from build123d import *

# Parameters (mm, degrees)
SKETCH1_W               = 8
SKETCH1_H               = 8
BOSS_EXTRUDE1_DEPTH     = 3
CUT_EXTRUDE1_DEPTH      = 12.704699911
CUT_EXTRUDE1_DEPTH_BACK = 12.704699911
CUT_EXTRUDE2_DEPTH      = 11
SKETCH4_R               = 1.8
CUT_EXTRUDE3_DEPTH      = 0.8
SKETCH5_W               = 8
SKETCH5_H               = 1
BOSS_EXTRUDE2_DEPTH     = 2
FILLET1_R               = 4
CUT_EXTRUDE4_DEPTH      = 0.4
CUT_EXTRUDE5_DEPTH      = 0.4


with BuildPart() as part:
    # Sketch1 → Boss-Extrude1 (new body)
    with BuildSketch(Plane(origin=(0, 0, 0), x_dir=(1, 0, 0), z_dir=(0, 1, 0))):
        with Locations((4, 4)):
            Rectangle(SKETCH1_W, SKETCH1_H)
    extrude(amount=BOSS_EXTRUDE1_DEPTH)

    # Sketch2 → Cut-Extrude1 (cut, two sides: drawn at the far end of the back side and taken through both)
    with BuildSketch(Plane.XY.offset(-CUT_EXTRUDE1_DEPTH_BACK)):
        Polygon((0, 0), (0.6, 3), (0, 3), align=None)
        Polygon((8, 0), (7.4, 3), (8, 3), align=None)
    extrude(amount=CUT_EXTRUDE1_DEPTH + CUT_EXTRUDE1_DEPTH_BACK, mode=Mode.SUBTRACT)

    # Sketch3 → Cut-Extrude2 (cut)
    with BuildSketch(Plane(origin=(0, 0, 0), x_dir=(0, 0, -1), z_dir=(1, 0, 0))):
        Polygon((0, 0), (0.6, 3), (0, 3), align=None)
        Polygon((8, 3), (7.4, 3), (8, 0), align=None)
    extrude(amount=CUT_EXTRUDE2_DEPTH, mode=Mode.SUBTRACT)

    # Sketch4 → Cut-Extrude3 (cut)
    with BuildSketch(Plane.XZ):
        with Locations(Location((4, -3.75, 0), (0, 0, 270))):
            Circle(SKETCH4_R)
    extrude(amount=-CUT_EXTRUDE3_DEPTH, mode=Mode.SUBTRACT)

    # Sketch5 → Boss-Extrude2 (add)
    with BuildSketch(Plane.XZ):
        with Locations((4, -7.5)):
            Rectangle(SKETCH5_W, SKETCH5_H)
    extrude(amount=BOSS_EXTRUDE2_DEPTH)

    # Fillet1
    # the kernel refuses this fillet: 4 mm, written as the material it takes off along each edge
    with BuildSketch(Plane(origin=(8, -2, -16.660254038), x_dir=(0, 1, 0), z_dir=(0, 0, 1)), Plane(origin=(0, -2, 1.660254038), x_dir=(0, 1, 0), z_dir=(0, 0, -1))) as fillet1_piece_1:
        with BuildLine():
            CenterArc((4, 3.464101615), FILLET1_R, 180, 60)
            Line((0, 3.464101615), (-0.08, 3.464101615))
            Line((-0.08, 3.464101615), (-0.08, 0))
            Line((-0.08, 0), (0, -0.08))
            ThreePointArc((0, -0.08), (1, -0.08), (1.96, -0.069282032))
            Line((1.96, -0.069282032), (2, 0))
        make_face()
    extrude(amount=18.320508076, mode=Mode.SUBTRACT)

    # Sketch6 → Cut-Extrude4 (cut)
    with BuildSketch(Plane(origin=(0, 3, 0), x_dir=(1, 0, 0), z_dir=(0, 1, 0))):
        Polygon((2.721575188, 1.941169366), (2.721575188, 5.941169366), (5.439523906, 5.941169366), (5.439523906, 5.2745027), (3.490805957, 5.2745027), (3.490805957, 4.300143725), (5.18311365, 4.300143725), (5.18311365, 3.633477059), (3.490805957, 3.633477059), (3.490805957, 1.941169366), align=None)
    extrude(amount=-CUT_EXTRUDE4_DEPTH, mode=Mode.SUBTRACT)

    # Sketch7 → Cut-Extrude5 (cut)
    with BuildSketch(Plane(origin=(0, 3, 0), x_dir=(1, 0, 0), z_dir=(0, 1, 0))):
        Polygon((6.374503362, 0.955347226), (6.374503362, 3.239962611), (7.020657208, 3.239962611), (7.020657208, 2.939962611), (6.720657208, 2.939962611), (6.720657208, 1.255347226), (7.020657208, 1.255347226), (7.020657208, 0.955347226), align=None)
    extrude(amount=-CUT_EXTRUDE5_DEPTH, mode=Mode.SUBTRACT)


solid = part.part
Design review of the part built by this model. Coordinates are the model's own, in mm. A direction names the side the tool comes from. Coordinates: 2 decimals unless noted, no trailing zeros. Loops run counter-clockwise (first coordinate to the right, second up) from the corner with the lowest first, then second, coordinate; pieces in that order, holes last. Notation, with made-up numbers: (73, 11) -> (117, 11) arc R17 cw to (117, 23) -> close; hole circle Ø3 at (-21, 48.5). An arc over 180 degrees is marked (long way). Use a Markdown table: item, result. Add a question column.
Item 1: We need section D-D, the plane y = 0.95. Write out the cut boundary in (x, z).
Item 2: Wall thickness on L1, parallel to Z at x = 4.5, y = -0.2; L2, parallel to X at y = 0.35, z = -3.75; L3, parallel to Y at x = 7, z = -6.5: over which ranges is each line inside the solid? List them lowest first. Write a range as from..to.
Item 3: Clearance check with flat-ended pins moving along their axes: P1, Ø1, axis at x = 2, y = 0.5, coming from the +Z side; P2, Ø1, axis at x = 4, y = -1, coming from the +Z side; P3, Ø3, axis at x = 4.5, z = -4, coming from the -Y side. State where each tip first meets the part, or that it passes through.
Item 4: The part is to be moulded in two halves that separate along X. For faces 1 (the flat face through (4, 0.8, -4)), 2 (the flat face through (0.3, 1.5, -4.1)), 3 (the flat face through (4, -1, -7)), say which applies: +X half, -X half, draft (parallel to the pull), parting line (faces both ways), or undercut.
Item 5: Machinability: for faces 4 (the cylindrical face through (4.541, 0.394, -5.467)), 5 (the flat face through (3, 0, -2)), 6 (the flat face through (4, -1, -8)), which of the approach directions +Z, -Z, +X, -X, +Y, -Y give a long, thin tool a straight path to every point of the face, cutting with its end or side? Answer none if there is none.
Item 6: We need section C-C, the plane z = -3.75. Write out the cut boundary in (x, y), and give its area (3 significant figures).
Item 7: We need section A-A, the plane x = 4. Write out the cut boundary in (y, z), and give its area (3 significant figures).
Item 8: We need section B-B, the plane y = 2.7. Write out the cut boundary in (x, z).
Numbers:
| question | item | result |
|---|---|---|
| 1 | outline | (0.19, -7.81) -> (7.81, -7.81) -> (7.81, -0.19) -> (0.19, -0.19) -> close |
| 2 | L1 | z = -8..-7 |
| 2 | L2 | x = 0.07..2.2, 5.8..7.93 |
| 2 | L3 | y = 0..3 |
| 3 | P1 | stops at z = 0 |
| 3 | P2 | stops at z = -7 |
| 3 | P3 | stops at y = 0 |
| 4 | face 1 | undercut |
| 4 | face 2 | -X half |
| 4 | face 3 | draft |
| 5 | face 4 | -Y |
| 5 | face 5 | +Z, +X, -X, -Y |
| 5 | face 6 | -Z, +X, -X, +Y, -Y |
| 6 | outline | (0, 0) -> (2.2, 0) -> (2.2, 0.8) -> (5.8, 0.8) -> (5.8, 0) -> (8, 0) -> (7.4, 3) -> (5.18, 3) -> (5.18, 2.6) -> (2.72, 2.6) -> (2.72, 3) -> (0.6, 3) -> close |
| 6 | area | 18.3 mm^2 |
| 7 | outline | (-2, -8) -> (0, -8) -> (3, -7.4) -> (3, -5.94) -> (2.6, -5.94) -> (2.6, -5.27) -> (3, -5.27) -> (3, -4.3) -> (2.6, -4.3) -> (2.6, -3.63) -> (3, -3.63) -> (3, -0.6) -> (0, 0) -> (0, -1.95) -> (0.8, -1.95) -> (0.8, -5.55) -> (0, -5.55) -> (0, -7) -> (-2, -7) -> close |
| 7 | area | 20.8 mm^2 |
| 8 | outline | (0.54, -7.46) -> (7.46, -7.46) -> (7.46, -0.54) -> (0.54, -0.54) -> close; hole (2.72, -5.94) -> (5.44, -5.94) -> (5.44, -5.27) -> (3.49, -5.27) -> (3.49, -4.3) -> (5.18, -4.3) -> (5.18, -3.63) -> (3.49, -3.63) -> (3.49, -1.94) -> (2.72, -1.94) -> close; hole (6.37, -3.24) -> (7.02, -3.24) -> (7.02, -2.94) -> (6.72, -2.94) -> (6.72, -1.26) -> (7.02, -1.26) -> (7.02, -0.96) -> (6.37, -0.96) -> close |
